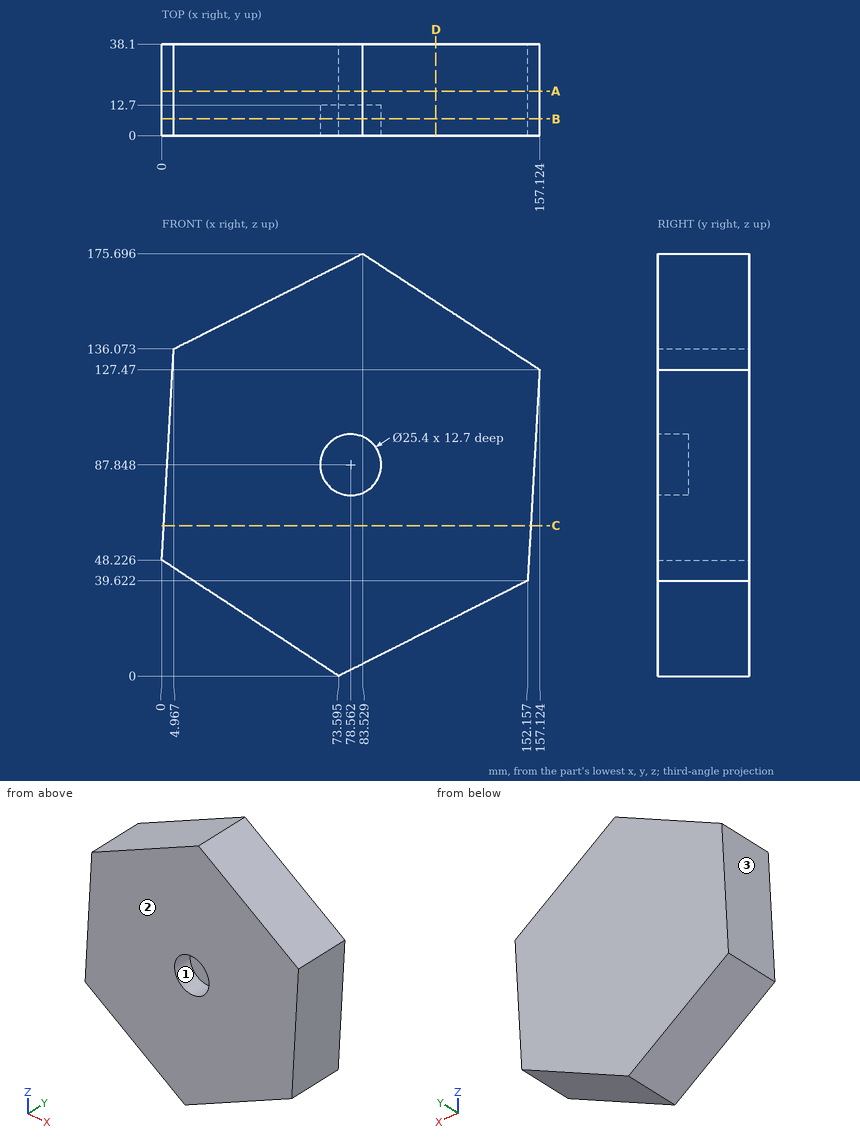
Source: three-view drawing plus pictorial views. Frame: mm from the lowest corner of the part. Coordinates: 2 decimals unless noted, no trailing zeros. Order: outer loops, then holes, each group sorted by start corner. A loop starts at its lowest first (then second) coordinate and runs counter-clockwise, first axis right, second up. Notation, with made-up numbers: M 9,-9 L 65,-9 A6 cw 65,2 Z; hole C 39,48 d6. An arc over 180 degrees is marked long. Write each question's results on one line, items separated by ' | '. Start each with the question number.
1. Section C-C, the plane z = 62.5. Return the cut outline in (x, y).
2. Pin query (flat end, axial travel): pin 1 (10 mm diameter, centred on x = 74.5, y = 4.5, fed in from +Z); pin 2 (3 mm diameter, centred on x = 41.5, y = 6.5, fed in from +Z) (1 decimal); pin 3 (2 mm diameter, centred on x = 84, y = 26.5, fed in from -Z); pin 4 (1 mm diameter, centred on x = 45.5, z = 157.5, fed in from -Y). Return the tip coordinate at first contact, or that it passes through.
3. Material intervals for L1, parallel to X at y = 32.5, z = 63 (1 decimal); L2, parallel to X at y = 30.5, z = 52; L3, parallel to Z at x = 35, y = 25, sorted ascending.
4. Section A-A, the plane y = 18.5. Return the cut outline in (x, z) (1 decimal), then the cut area to 3 significant figures.
5. Section B-B, the plane y = 7. Return the cut outline in (x, z) (1 decimal), then the cut area to 3 significant figures.
6. Section D-D, the plane x = 114. Return the cut outline in (y, z).
7. Draft query along X for the marked faces 1, 2 and 3. Return one class per face: +X half, -X half, draft (parallel to the pull), parting line (faces both ways), or undercut.
Solution:
1) outline: M 0.81,0 L 153.45,0 L 153.45,38.1 L 0.81,38.1 Z
2) pin 1: z = 173.66 | pin 2: z = 155.3 | pin 3: z = 4.74 | pin 4: through
3) L1: 0.8 to 153.5 | L2: 0.21 to 152.86 | L3: 25.29 to 151.22
4) outline: M 0,48.2 L 73.6,0 L 152.2,39.6 L 157.1,127.5 L 83.5,175.7 L 5,136.1 Z | area: 20,100 mm²
5) outline: M 0,48.2 L 73.6,0 L 152.2,39.6 L 157.1,127.5 L 83.5,175.7 L 5,136.1 Z; hole C 78.6,87.8 d25.4 | area: 19,600 mm²
6) outline: M 0,20.38 L 38.1,20.38 L 38.1,155.73 L 0,155.73 Z
7) face 1: undercut | face 2: draft | face 3: -X half
